Input: part model. Units: mm. Frame: model coordinates. A direction names the side the tool comes from. Give positions to 0.01 mm unless a question says otherwise; leave off trailing zeros. Loops run counter-clockwise (first coordinate to the right, second up) from the corner with the lowest first, then second, coordinate; pieces in that order, holes last. Notation, with made-up numbers: (71, 55) -> (85, 55) arc R10 ccw to (85, 64) -> close; hole circle Ø10 at (65, -26). An arc over 180 degrees is marked (long way). Answer in a Markdown table with one row per item. Add a question column.
```python
from build123d import *

# Parameters (mm, degrees)
SKETCH2_R                    = 10
CUT_EXTRUDE1_DEPTH           = 230.761019694
M24_TAPPED_HOLE1_D           = 21
M24_TAPPED_HOLE1_DEPTH       = 27
M24_TAPPED_HOLE1_CSINK_D     = 24.05
M24_TAPPED_HOLE1_CSINK_ANGLE = 90
M24_TAPPED_HOLE1_TIP         = 6.3090365
M12_TAPPED_HOLE1_D           = 10.2
M12_TAPPED_HOLE1_DEPTH       = 17.25
M12_TAPPED_HOLE1_CSINK_D     = 12.05
M12_TAPPED_HOLE1_CSINK_ANGLE = 90
M12_TAPPED_HOLE1_TIP         = 3.064389157


with BuildPart() as part:
    # Sketch1 → Revolve1 (revolve)
    with BuildSketch(Plane.XY, mode=Mode.PRIVATE) as revolve1_sk:
        with BuildLine():
            Line((5.306451613, -6.774193548), (-15.693548387, -6.774193548))
            Line((-15.693548387, -6.774193548), (-15.693548387, 10.142902683))
            Line((-15.693548387, 10.142902683), (-1.693548387, 18.225806452))
            Line((-1.693548387, 18.225806452), (-1.693548387, 74.225806452))
            Line((-1.693548387, 74.225806452), (58.306451613, 74.225806452))
            ThreePointArc((58.306451613, 74.225806452), (60.063810926, 69.983165764), (64.306451613, 68.225806452))
            Line((64.306451613, 68.225806452), (108.306451613, 68.225806452))
            Line((108.306451613, 68.225806452), (108.306451613, 46.225806452))
            Line((108.306451613, 46.225806452), (51.306451613, 46.225806452))
            Line((51.306451613, 46.225806452), (51.306451613, 40.225806452))
            Line((51.306451613, 40.225806452), (5.306451613, -6.774193548))
        make_face()
    revolve(revolve1_sk.sketch.rotate(Axis((-29.693548387, 26.362903226, 0), (0, -1, 0)), 180), axis=Axis((-29.693548387, 26.362903226, 0), (0, -1, 0)))

    # Sketch2 → Cut-Extrude1 (cut, through all)
    with BuildSketch(Plane(origin=(0, 68.225806452, 0), x_dir=(1, 0, 0), z_dir=(0, 1, 0))):
        with Locations(Location((-29.693548387, 112.5, 0), (0, 0, 180))):
            Circle(SKETCH2_R)
        with Locations(Location((67.734309539, 56.25, 0), (0, 0, 180))):
            Circle(SKETCH2_R)
        with Locations(Location((67.734309539, -56.25, 0), (0, 0, 180))):
            Circle(SKETCH2_R)
        with Locations(Location((-29.693548387, -112.5, 0), (0, 0, 180))):
            Circle(SKETCH2_R)
        with Locations(Location((-127.121406313, -56.25, 0), (0, 0, 180))):
            Circle(SKETCH2_R)
        with Locations(Location((-127.121406313, 56.25, 0), (0, 0, 180))):
            Circle(SKETCH2_R)
    extrude(amount=-CUT_EXTRUDE1_DEPTH, mode=Mode.SUBTRACT)

    # M24 Tapped Hole1
    with Locations(Plane(origin=(0, 74.225806452, 0), x_dir=(1, 0, 0), z_dir=(0, 1, 0))):
        with Locations((-29.693548387, 60), (-29.693548387, -60)):
            CounterSinkHole(M24_TAPPED_HOLE1_D / 2, M24_TAPPED_HOLE1_CSINK_D / 2, depth=M24_TAPPED_HOLE1_DEPTH, counter_sink_angle=M24_TAPPED_HOLE1_CSINK_ANGLE)
            with Locations((0, 0, -(M24_TAPPED_HOLE1_DEPTH + M24_TAPPED_HOLE1_TIP / 2))):  # 118° drill point
                Cone(0, M24_TAPPED_HOLE1_D / 2, M24_TAPPED_HOLE1_TIP, mode=Mode.SUBTRACT)

    # M12 Tapped Hole1
    with Locations(Plane(origin=(0, 74.225806452, 0), x_dir=(1, 0, 0), z_dir=(0, 1, 0))):
        with Locations((14.306451613, 0), (-73.693548387, 0)):
            CounterSinkHole(M12_TAPPED_HOLE1_D / 2, M12_TAPPED_HOLE1_CSINK_D / 2, depth=M12_TAPPED_HOLE1_DEPTH, counter_sink_angle=M12_TAPPED_HOLE1_CSINK_ANGLE)
            with Locations((0, 0, -(M12_TAPPED_HOLE1_DEPTH + M12_TAPPED_HOLE1_TIP / 2))):  # 118° drill point
                Cone(0, M12_TAPPED_HOLE1_D / 2, M12_TAPPED_HOLE1_TIP, mode=Mode.SUBTRACT)


solid = part.part
```
1) Section A-A on y = 61. State how many separate pieces and enclosed holes the cut face has, and give its area (3 significant figures).
2) Pull-direction query (Z, two-part tool) for faces 4 (the face through (-68.6, 65.02, -0.22)), 5 (the face through (72.018, 57.072, -93.267)), 6 (the face through (-50, 74.226, -21)); classes: +Z half, -Z half, draft (parallel to the pull), parting line (faces both ways), or undercut.
3) Material intervals for line 1 along X through (y, z) = (62, -56); line 2 along X through (y, z) = (63, -60); line 3 along Y through (x, z) = (-139, -73), sorted ascending.
4) Section D-D on y = 29.5. Output: boundary loops of the cut face in (x, z).
5) Section B-B on z = -112.5. Output: boundary loops of the cut face in (x, y).
6) Reachability of faces 1 (the face through (-106.953, 43.184, -24.33)), 2 (the face through (18.354, 65.024, 3.103)), 3 (the face through (-42.626, 1.803, 5.362)) from +Z, -Z, +X, -X, +Y, -Y: full face, straight path, thin tool, end or side. Return the list, or none.
7) Pin query (flat end, axial travel): pin 1 (3 mm diameter, centred on x = -38, y = 2.5, fed in from +Z); pin 2 (1 mm diameter, centred on x = -42.5, y = 12.5, fed in from +Z); pin 3 (12 mm diameter, centred on y = 63, z = 70, fed in from +X). Return the tip coordinate at first contact, or that it passes through.
Working result:
| question | item | result |
|---|---|---|
| 1 | separate pieces | 1 |
| 1 | enclosed holes | 11 |
| 1 | area | 54,600 mm2 |
| 2 | face 4 | undercut |
| 2 | face 5 | parting line |
| 2 | face 6 | draft |
| 3 | line 1 | x = -155.82 to -137.12, -117.12 to -39.4, -19.99 to 57.74, 77.73 to 96.43 |
| 3 | line 2 | x = -153.97 to -136.39, -117.85 to -40.19, -19.19 to 58.46, 77 to 94.58 |
| 3 | line 3 | y = 46.23 to 68.23 |
| 4 | outline | circle Ø141 at (-29.69, 0); hole circle Ø56 at (-29.69, 0) |
| 5 | outline | (-109.62, 46.23) -> (-39.69, 46.23) -> (-39.69, 68.23) -> (-109.62, 68.23) -> close; (-19.69, 46.23) -> (50.23, 46.23) -> (50.23, 68.23) -> (-19.69, 68.23) -> close |
| 6 | face 1 | -Y |
| 6 | face 2 | +Y |
| 6 | face 3 | +Y, -Y |
| 7 | pin 1 | stops at z = 44.81 |
| 7 | pin 2 | stops at z = 52.84 |
| 7 | pin 3 | stops at x = 92.57 |
